from build123d import *

# Parameters (mm, degrees)
SKETCH_1_W      = 1800
SKETCH_1_H      = 750
EXTRUDE_1_DEPTH = 40
SKETCH_2_W      = 50
SKETCH_2_H      = 50
EXTRUDE_2_DEPTH = 700
SKETCH_3_W      = 50
SKETCH_3_H      = 550
SKETCH_3_W_2    = 1600
SKETCH_3_H_2    = 50
EXTRUDE_3_DEPTH = 80
EXTRUDE_4_REACH = 2039.768
SKETCH_4_W      = 50
SKETCH_4_H      = 50
EXTRUDE_5_REACH = 1987.573
SKETCH_5_W      = 100
SKETCH_5_H      = 50


with BuildPart() as part:
    # ｽｹｯﾁ1 → ﾎﾞｽ - 押し出し1 (new body)
    with BuildSketch(Plane(origin=(0, 0, 0), x_dir=(1, 0, 0), z_dir=(0, 1, 0))):
        with Locations((900, 375)):
            Rectangle(SKETCH_1_W, SKETCH_1_H)
    extrude(amount=EXTRUDE_1_DEPTH)

    # ｽｹｯﾁ2 → ﾎﾞｽ - 押し出し2 (add)
    with BuildSketch(Plane(origin=(0, 0, 0), x_dir=(-1, 0, 0), z_dir=(0, -1, 0))):
        with Locations((-1725, 75)):
            Rectangle(SKETCH_2_W, SKETCH_2_H)
        with Locations((-1725, 675)):
            Rectangle(SKETCH_2_W, SKETCH_2_H)
        with Locations((-75, 75)):
            Rectangle(SKETCH_2_W, SKETCH_2_H)
        with Locations((-75, 675)):
            Rectangle(SKETCH_2_W, SKETCH_2_H)
    extrude(amount=EXTRUDE_2_DEPTH)

    # ｽｹｯﾁ3 → ﾎﾞｽ - 押し出し3 (add)
    with BuildSketch(Plane(origin=(0, 0, 0), x_dir=(-1, 0, 0), z_dir=(0, -1, 0))):
        with Locations((-1725, 375)):
            Rectangle(SKETCH_3_W, SKETCH_3_H)
        with Locations((-900, 675)):
            Rectangle(SKETCH_3_W_2, SKETCH_3_H_2)
        with Locations((-900, 75)):
            Rectangle(SKETCH_3_W_2, SKETCH_3_H_2)
        with Locations((-75, 375)):
            Rectangle(SKETCH_3_W, SKETCH_3_H)
    extrude(amount=EXTRUDE_3_DEPTH)

    # ｽｹｯﾁ4 → ﾎﾞｽ - 押し出し4 (add, up to next)
    with BuildSketch(Plane.XY.offset(-650), mode=Mode.PRIVATE) as extrude_4_sk1:
        with Locations((1725, -615)):
            Rectangle(SKETCH_4_W, SKETCH_4_H)
    extrude_4_tool1 = extrude(extrude_4_sk1.sketch, amount=EXTRUDE_4_REACH, mode=Mode.PRIVATE) - part.part
    # ｽｹｯﾁ4 → ﾎﾞｽ - 押し出し4 (add, up to next)
    with BuildSketch(Plane.XY.offset(-650), mode=Mode.PRIVATE) as extrude_4_sk2:
        with Locations((75, -615)):
            Rectangle(SKETCH_4_W, SKETCH_4_H)
    extrude_4_tool2 = extrude(extrude_4_sk2.sketch, amount=EXTRUDE_4_REACH, mode=Mode.PRIVATE) - part.part
    add(extrude_4_tool1.solids().sort_by_distance((1725, -615, -650))[0])
    add(extrude_4_tool2.solids().sort_by_distance((75, -615, -650))[0])

    # ｽｹｯﾁ5 → ﾎﾞｽ - 押し出し5 (add, up to next)
    with BuildSketch(Plane.ZY.offset(-1700), mode=Mode.PRIVATE) as extrude_5_sk1:
        with Locations((-375, -615)):
            Rectangle(SKETCH_5_W, SKETCH_5_H)
    extrude_5_tool1 = extrude(extrude_5_sk1.sketch, amount=EXTRUDE_5_REACH, mode=Mode.PRIVATE) - part.part
    add(extrude_5_tool1.solids().sort_by_distance((1700, -615, -375))[0])


solid = part.part
Design review of the part built by this model. Coordinates are the model's own, in mm. A direction names the side the tool comes from. Round coordinates to 2 decimals unless told otherwise and drop trailing zeros. Order: outer loops, then holes, each group sorted by start corner. A loop starts at its lowest first (then second) coordinate and runs counter-clockwise, first axis right, second up. Notation, with made-up numbers: M -35,38 L -21,38 A30 cw -21,70 Z; hole C 50,-13.75 d6. An arc over 180 degrees is marked long. Answer as CSV lines item,"result". Start each with the question number.
1) Add section D-D (z = -683). Give the boundary of the cut face in (x, y), then the cut area to 3 significant figures.
2) Tool access review of faces 4 (the face through (904, -63, -700)), 5 (the face through (911, -39, -100)), 6 (the face through (75, -670, -100)), 7 (the face through (100, -457, -654)), 8 (the face through (75, -331, -650)): name each direction out of +Z, -Z, +X, -X, +Y, -Y from which nothing blocks a thin tool from reaching the whole face with its end or side.
3) The part is to be moulded in two halves that separate along Z. For faces 1 (the face through (1725, -670, -650)), 2 (the face through (1800, 20, -370)), 3 (the face through (904, -63, -50)), say which applies: +Z half, -Z half, draft (parallel to the pull), parting line (faces both ways), or undercut.
4) Add section C-C (z = -369). Give the boundary of the cut face in (x, y), then the cut area to 3 significant figures.
5) Add section A-A (y = -394.5). Give the boundary of the cut face in (x, z).
6) Wall thickness on line 1 along X through (y, z) = (-21.5, -550); line 2 along Z through (x, y) = (84, -151); line 3 along Y through (x, z) = (311, -588): over which ranges is each line inside the solid? List them lowest first. Write a range as [from, to].
7) For pin 1 Ø1.5 at (x, y) = (1205.5, -616) entering from -Z; pin 2 Ø8 at (x, z) = (247.5, -158) entering from -Y; pin 3 Ø15 at (x, z) = (866.5, -670.5) entering from -Y, all flat-tipped, find the tip position at first contact; note any pin that passes through.
8) Add section B-B (x = 136). Give the boundary of the cut face in (y, z).
Resolved:
1,outline,"M 0,0 L 50,0 L 50,-700 L 100,-700 L 100,-80 L 1700,-80 L 1700,-700 L 1750,-700 L 1750,0 L 1800,0 L 1800,40 L 0,40 Z"
1,area,"270,000 mm^2"
2,face 4,"-Z, +X, -X, -Y"
2,face 5,"-Y"
2,face 6,"+X, -X, -Y"
2,face 7,"-Z, -Y"
2,face 8,"+X, -X"
3,face 1,"undercut"
3,face 2,"draft"
3,face 3,"+Z half"
4,outline,"M 0,0 L 50,0 L 50,-80 L 100,-80 L 100,0 L 1700,0 L 1700,-80 L 1750,-80 L 1750,0 L 1800,0 L 1800,40 L 0,40 Z; M 50,-640 L 1750,-640 L 1750,-590 L 50,-590 Z"
4,area,"165,000 mm^2"
5,outline,"M 50,-700 L 100,-700 L 100,-650 L 50,-650 Z; M 50,-100 L 100,-100 L 100,-50 L 50,-50 Z; M 1700,-700 L 1750,-700 L 1750,-650 L 1700,-650 Z; M 1700,-100 L 1750,-100 L 1750,-50 L 1700,-50 Z"
6,line 1,"[50, 100], [1700, 1750]"
6,line 2,"[-700, -650], [-100, -50]"
6,line 3,"[0, 40]"
7,pin 1,"z = -425"
7,pin 2,"y = 0"
7,pin 3,"y = -80"
8,outline,"M -640,-425 L -590,-425 L -590,-325 L -640,-325 Z; M -80,-700 L 0,-700 L 0,-750 L 40,-750 L 40,0 L 0,0 L 0,-50 L -80,-50 L -80,-100 L 0,-100 L 0,-650 L -80,-650 Z"
